The figure shows three views and two pictorial views of one solid part (mm, origin at its lowest corner). Answer the questions. Give positions to 0.01 mm unless a question says otherwise; leave off trailing zeros. Loops run counter-clockwise (first coordinate to the right, second up) from the corner with the lowest first, then second, coordinate; pieces in that order, holes last. Notation, with made-up numbers: (22.25, -0.5) - (54.25, -0.5) arc R13 ccw to (54.25, 12.5) - close; hole circle Ø5 at (-10, 60). An arc over 180 degrees is marked (long way). Use CSV: the item, a comma, the result in double quotes.
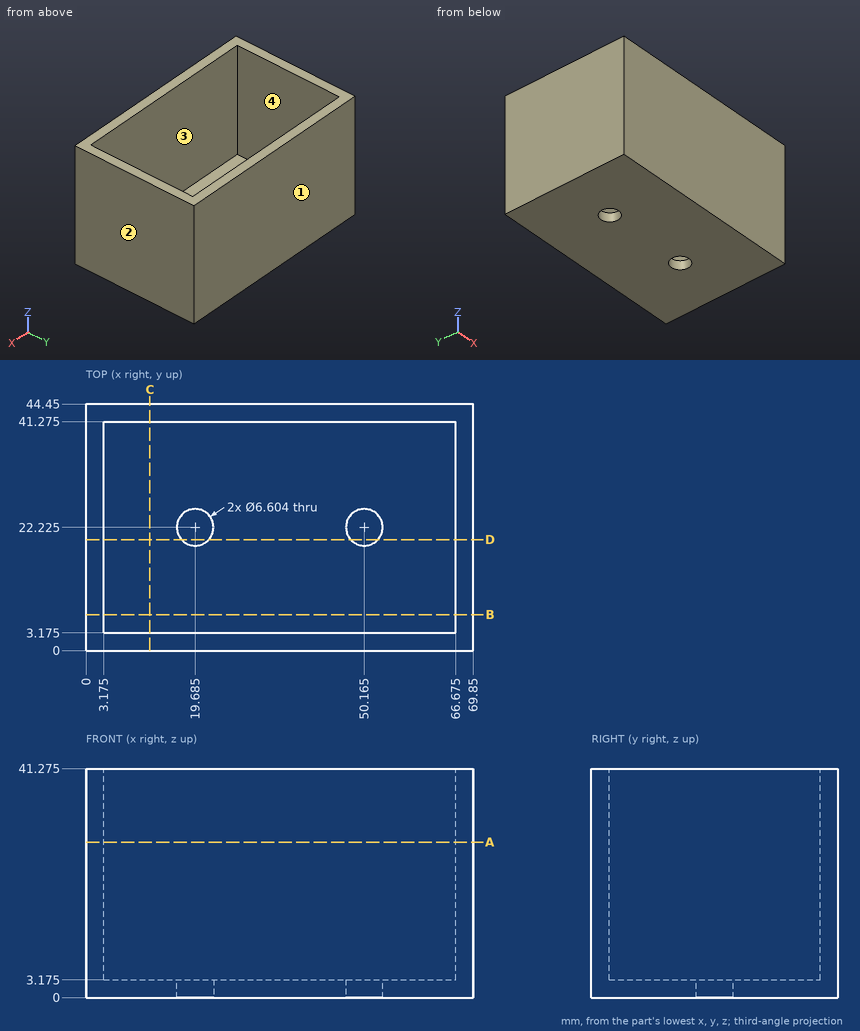
Item 1: A cutting plane is placed at B-B on y = 6.5. Determine the outline of the cut face in (x, z) (3 decimals), and give its area (3 significant figures).
Determined:
outline,"(0, 0) - (69.85, 0) - (69.85, 41.275) - (66.675, 41.275) - (66.675, 3.175) - (3.175, 3.175) - (3.175, 41.275) - (0, 41.275) - close"
area,"464 mm²"
Item 2: Find the intervals of material crossed by line 1 (Y direction, x = 35, z = 26.5) (3 decimals); line 2 (X direction, y = 22.5, z = 17.5) (3 decimals); line 3 (Z direction, x = 29.5, y = 41) (3 decimals), in increasing order.
Determined:
line 1,"y = 0 to 3.175, 41.275 to 44.45"
line 2,"x = 0 to 3.175, 66.675 to 69.85"
line 3,"z = 0 to 3.175"
Item 3: The mould has two halves that part along Y. Classify the marked faces 1, 2, 3 and 4: pulls with the +Y half, pulls with the -Y half, needs draft (parallel to the pull), parting line crosses it, or undercut.
Determined:
face 1,"pulls with the +Y half"
face 2,"needs draft"
face 3,"undercut"
face 4,"undercut"
Item 4: A cutting plane is placed at D-D on y = 20. Determine the outline of the cut face in (x, z) (3 decimals), and give its area (3 significant figures).
Determined:
outline,"(0, 0) - (17.245, 0) - (17.245, 3.175) - (3.175, 3.175) - (3.175, 41.275) - (0, 41.275) - close; (22.125, 0) - (47.725, 0) - (47.725, 3.175) - (22.125, 3.175) - close; (52.605, 0) - (69.85, 0) - (69.85, 41.275) - (66.675, 41.275) - (66.675, 3.175) - (52.605, 3.175) - close"
area,"433 mm²"
Item 5: Given P1, Ø10.5, axis at x = 50.165, y = 22.225, coming from the +Z side (3 decimals); P2, Ø10, axis at y = 23.5, z = 11.5, coming from the -X side, each flat-ended and moving along its own axis, determine where each tip first touches the part or whether it passes through.
Determined:
P1,"stops at z = 3.175"
P2,"stops at x = 0"
Item 6: A cutting plane is placed at A-A on z = 28. Determine the outline of the cut face in (x, y) (3 decimals).
Determined:
outline,"(0, 0) - (69.85, 0) - (69.85, 44.45) - (0, 44.45) - close; hole (3.175, 3.175) - (66.675, 3.175) - (66.675, 41.275) - (3.175, 41.275) - close"
Item 7: A cutting plane is placed at C-C on x = 11.5. Determine the outline of the cut face in (y, z) (3 decimals).
Determined:
outline,"(0, 0) - (44.45, 0) - (44.45, 41.275) - (41.275, 41.275) - (41.275, 3.175) - (3.175, 3.175) - (3.175, 41.275) - (0, 41.275) - close"
